from build123d import *

# Parameters (mm, degrees)
SKETCH3_W                = 11
SKETCH3_H                = 21
BOSS_EXTRUDE1_DEPTH      = 10
CUT_EXTRUDE1_DEPTH       = 8
CUT_EXTRUDE5_DEPTH       = 8
CUT_EXTRUDE5_DEPTH_BACK  = 8
BOSS_EXTRUDE2_DEPTH      = 5.5
BOSS_EXTRUDE2_DEPTH_BACK = 5.5
BOSS_EXTRUDE6_DEPTH      = 120
CUT_EXTRUDE6_DEPTH       = 120


with BuildPart() as part:
    # Sketch3 → Boss-Extrude1 (new body)
    with BuildSketch(Plane.XY):
        Rectangle(SKETCH3_W, SKETCH3_H)
    extrude(amount=BOSS_EXTRUDE1_DEPTH)

    # Sketch5 → Cut-Extrude1 (cut)
    with BuildSketch(Plane.XY):
        Polygon((0, 1.5), (-2, 1.5), (-2, -1.5), (2, -1.5), (2, 1.5), align=None)
    extrude(amount=CUT_EXTRUDE1_DEPTH, mode=Mode.SUBTRACT)

    # Sketch6 → Cut-Extrude5 (cut, two sides: drawn at the far end of the back side and taken through both)
    with BuildSketch(Plane(origin=(0, 0, 0), x_dir=(0, 0, -1), z_dir=(1, 0, 0)).offset(-CUT_EXTRUDE5_DEPTH_BACK)):
        Polygon((-1.0867085, -10.5), (-6.011599163, -7.693477847), (-8.753565317, 0), (-10, 10.5), (-10, -10.5), (-10, -11.324459918), (-1.0867085, -10.760658811), align=None)
    extrude(amount=CUT_EXTRUDE5_DEPTH + CUT_EXTRUDE5_DEPTH_BACK, mode=Mode.SUBTRACT)

    # Sketch18 → Boss-Extrude2 (add, two sides: drawn at the far end of the back side and taken through both)
    with BuildSketch(Plane(origin=(0, 0, 0), x_dir=(0, 0, -1), z_dir=(1, 0, 0)).offset(-BOSS_EXTRUDE2_DEPTH_BACK)):
        Polygon((0, 10.5), (47.274579224, 275.316482995), (37.430212914, 277.073882193), (-10, 10.5), align=None)
    extrude(amount=BOSS_EXTRUDE2_DEPTH + BOSS_EXTRUDE2_DEPTH_BACK)

    # Sketch20 → Boss-Extrude6 (add)
    with BuildSketch(Plane(origin=(0, 274.99219554, -49.091129779), x_dir=(1, 0, 0), z_dir=(0, 0.9844366310526066, -0.17573991988673054))):
        Polygon((5.5, -11.845269159), (89.722424634, 9.543427454), (126.59891896, 25.507030725), (124.938057952, 30.22777974), (87.652020554, 14.094628059), (5.5, -6.845269159), (-5.5, -6.845269159), (-87.652020554, 14.094628059), (-124.938057952, 30.22777974), (-126.59891896, 25.507030725), (-89.722424634, 9.543427454), (-5.5, -11.845269159), align=None)
    extrude(amount=BOSS_EXTRUDE6_DEPTH)

    # Sketch23 → Cut-Extrude6 (cut)
    with BuildSketch(Plane(origin=(0, 3.839085852, 21.505283175), x_dir=(1, 0, 0), z_dir=(0, 0.17573991988673054, 0.9844366310526066))):
        Polygon((-5.5, 419.339661758), (-1.559239103, 421.572876694), (-44.351514871, 435.559129211), (-45.770075722, 435.559129211), (-131.689368664, 409.111534998), (-185.542931008, 339.339661758), (-131.689368664, 359.582766362), (-121.100925347, 374.450322533), (-99.48017922, 390.223948639), (-79.722424634, 399.339661758), align=None)
        Polygon((5.5, 419.339661758), (79.722424634, 399.339661758), (99.48017922, 390.223948639), (121.100925347, 374.450322533), (131.689368664, 359.582766362), (185.542931008, 339.339661758), (131.689368664, 409.111534998), (45.770075722, 435.559129211), (44.351514871, 435.559129211), (1.559239103, 421.572876694), align=None)
    extrude(amount=-CUT_EXTRUDE6_DEPTH, mode=Mode.SUBTRACT)


solid = part.part
The listing builds one solid part. Answer for the finished solid, in the listing's coordinates (mm). A direction names the side the tool comes from. Give positions to 0.01 mm unless a question says otherwise; leave off trailing zeros. Write each loop counter-clockwise with the first axis right and the second up, starting at its lowest first coordinate (ties: lowest second). Pieces come first, ordered by that corner, then holes. Notation, with made-up numbers: (23, 81.5) - (37, 81.5) arc R12 cw to (37, 93.5) - close; hole circle Ø10 at (61, 35). An arc over 180 degrees is marked (long way). Use a Markdown table: item, result.
1. Section A-A on y = 325.5 is taken. Write down the section's boundary in (x, z), plus the area to 3 significant figures.
Values follow:
| item | result |
|---|---|
| outline | (-126.6, -84.02) - (-124.94, -88.81) - (-87.65, -72.43) - (-5.5, -51.15) - (5.5, -51.15) - (87.65, -72.43) - (124.94, -88.81) - (126.6, -84.02) - (89.72, -67.8) - (5.5, -46.08) - (-5.5, -46.08) - (-89.72, -67.8) - close |
| area | 1,320 mm² |
2. Each of these flat-tipped pins is pushed along its axis until it touches: P1, Ø1.5, axis at y = 0, z = 6, coming from the +X side; P2, Ø10, axis at x = 52, z = -65.5, coming from the +Y side; P3, Ø1, axis at x = 88.5, y = 335, coming from the +Z side; P4, Ø17, axis at y = 180.5, z = -11.5, coming from the +X side. Where does it stop, or does it pass through?
Values follow:
| item | result |
|---|---|
| P1 | stops at x = 5.5 |
| P2 | stops at y = 393.27 |
| P3 | stops at z = -69.03 |
| P4 | passes through |
3. For a pull along X with two mould halves and no side action, classify faces 4 (the flat face through (106.56, 327.54, -81.1)), 5 (the flat face through (0.08, 334.43, -52.75)), 6 (the flat face through (-110.442, 372.576, -87.909)), 7 (the flat face through (107.9, 327.93, -76.23)) as released by +X, released by -X, zero draft, split by the parting line, or undercut.
Values follow:
| item | result |
|---|---|
| face 4 | undercut |
| face 5 | undercut |
| face 6 | released by -X |
| face 7 | released by +X |
4. Section C-C on z = -4.5 is taken. Write down the section's boundary in (x, y), plus the area to 3 significant figures.
Values follow:
| item | result |
|---|---|
| outline | (-5.5, 35.71) - (5.5, 35.71) - (5.5, 91.99) - (-5.5, 91.99) - close |
| area | 619 mm² |
5. Find the intervals of material crossed by probe 1 along X at (y, z) = (326.5, -79); probe 2 along X at (y, z) = (82.5, -6); probe 3 along X at (y, z) = (347.5, -85.5), in increasing order. Write a range as from..to.
Values follow:
| item | result |
|---|---|
| probe 1 | x = -114.78..-102.2, 102.2..114.78 |
| probe 2 | x = -5.5..5.5 |
| probe 3 | x = -121.04..-108.46, 108.46..121.04 |
6. A tool of negligible diameter and unlimited length cuts with its end or side. For faces 1 (the flat face through (0, 2, 0)), 2 (the flat face through (-106.034, 327.581, -80.876)), 3 (the flat face through (-66.332, 273.634, -56.702)), from which of +Z, -Z, +X, -X, +Y, -Y can it reach the whole face along a straight path? Write none if from no direction.
Values follow:
| item | result |
|---|---|
| face 1 | -Z, +X, -X, -Y |
| face 2 | -Z, -Y |
| face 3 | +Z, -X, -Y |
7. Section B-B on x = -25 is taken. Write down the section's boundary in (y, z), plus the area to 3 significant figures.
Values follow:
| item | result |
|---|---|
| outline | (275.32, -47.25) - (393.45, -68.33) - (394.34, -63.39) - (276.2, -42.31) - close |
| area | 602 mm² |
